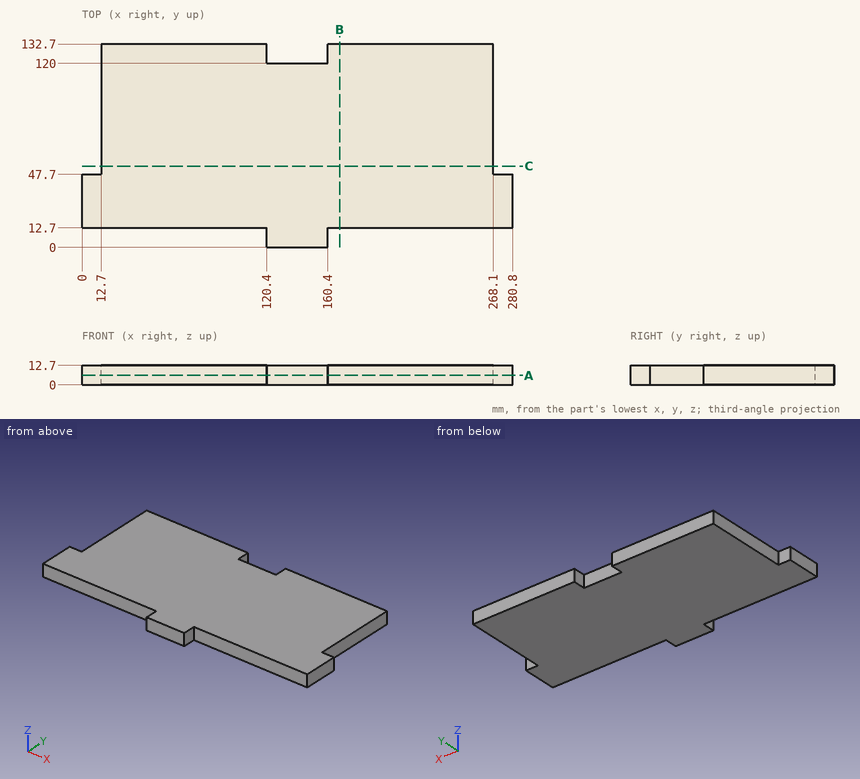
The figure shows three views and two pictorial views of one solid part (mm, origin at its lowest corner). Answer the questions. Give positions to 0.01 mm unless a question says otherwise; leave off trailing zeros. Loops run counter-clockwise (first coordinate to the right, second up) from the corner with the lowest first, then second, coordinate; pieces in that order, holes last. Notation, with made-up numbers: (28, -33.75) - (76, -33.75) arc R24 ccw to (76, -21.75) - close; hole circle Ø8 at (-34.5, 45.25). An arc over 180 degrees is marked (long way). Answer in a Markdown table with one row per item.
(1) Section A-A (z = 6.25) is taken. Give the vertices of the cut face in (x, y), and give its area (3 significant figures).
Results list:
| item | result |
|---|---|
| outline | (0, 12.7) - (120.4, 12.7) - (120.4, 0) - (160.4, 0) - (160.4, 12.7) - (280.8, 12.7) - (280.8, 47.7) - (268.1, 47.7) - (268.1, 132.7) - (160.4, 132.7) - (160.4, 120) - (120.4, 120) - (120.4, 132.7) - (12.7, 132.7) - (12.7, 47.7) - (0, 47.7) - close |
| area | 31,500 mm² |
(2) Section B-B (x = 168) is taken. Give the vertices of the cut face in (y, z).
Results list:
| item | result |
|---|---|
| outline | (12.7, 0) - (132.7, 0) - (132.7, 12.7) - (12.7, 12.7) - close |
(3) Flat-ended cylindrical pins translate along their axes: pin 1 Ø6.5 at (x, z) = (149.5, 8) entering from +Y; pin 2 Ø4 at (y, z) = (9, 5.5) entering from +X; pin 3 Ø4 at (y, z) = (125, 7.5) entering from +X. Find the tip coordinate at first contact, or state that the pin passes through.
Results list:
| item | result |
|---|---|
| pin 1 | stops at y = 120 |
| pin 2 | stops at x = 160.4 |
| pin 3 | stops at x = 268.1 |
(4) Section C-C (y = 53) is taken. Give the vertices of the cut face in (x, z).
Results list:
| item | result |
|---|---|
| outline | (12.7, 0) - (268.1, 0) - (268.1, 12.7) - (12.7, 12.7) - close |
(5) Consider L1, parallel to Y at x = 35, z = 11.5; L2, parallel to X at y = 64, z = 8; L3, parallel to X at y = 12.5, z = 9.5. Determine where each line is inside the solid, lowest interval first. Write a range as [from, to].
Results list:
| item | result |
|---|---|
| L1 | y = [12.7, 132.7] |
| L2 | x = [12.7, 268.1] |
| L3 | x = [120.4, 160.4] |
